Can you work these out from the model? Positions are in its coordinate system, mm. A direction names the side the tool comes from. Give positions to 0.01 mm unless a question says otherwise; leave off trailing zeros. Loops run counter-clockwise (first coordinate to the right, second up) from the corner with the lowest first, then second, coordinate; pieces in that order, holes last. Notation, with made-up numbers: M 73.25,6 L 115.25,6 A25 cw 115.25,26 Z; hole C -13,-23.5 d6. An arc over 180 degrees is marked long. Answer as a JSON object with one key per item and string values.
```python
from build123d import *

# Parameters (mm, degrees)
CROQUIS1_W                = 30
CROQUIS1_H                = 30
SALIENTE_EXTRUIR1_DEPTH   = 3
CROQUIS2_W                = 15
CROQUIS2_H                = 30
SALIENTE_EXTRUIR3_DEPTH   = 3
SALIENTE_EXTRUIR3_2_DEPTH = 3
CROQUIS3_W                = 30
CROQUIS3_H                = 30
SALIENTE_EXTRUIR4_DEPTH   = 3
SALIENTE_EXTRUIR5_DEPTH   = 3
CORTAR_EXTRUIR1_DEPTH     = 6
SALIENTE_EXTRUIR8_DEPTH   = 11
CROQUIS7_W                = 30
CROQUIS7_H                = 3.175
CORTAR_EXTRUIR3_DEPTH     = 18.542
CROQUIS9_W                = 60
CROQUIS9_H                = 0.175
SALIENTE_EXTRUIR9_DEPTH   = 11
CROQUIS10_W               = 90
CROQUIS10_H               = 5
CORTAR_EXTRUIR5_DEPTH     = 93
CROQUIS11_W               = 30
CROQUIS11_H               = 3.175
SALIENTE_EXTRUIR10_DEPTH  = 11
CROQUIS12_W               = 60
CROQUIS12_H               = 0.175
CORTAR_EXTRUIR6_DEPTH     = 11
CROQUIS14_W               = 30
CROQUIS14_H               = 6.35
CORTAR_EXTRUIR8_DEPTH     = 19.812
CROQUIS15_W               = 60
CROQUIS15_H               = 6.315381445
SALIENTE_EXTRUIR14_DEPTH  = 6
CROQUIS16_W               = 6.35
CROQUIS16_H               = 30
CORTAR_EXTRUIR9_DEPTH     = 10
CROQUIS17_W               = 3.35
CROQUIS17_H               = 60
SALIENTE_EXTRUIR15_DEPTH  = 6


with BuildPart() as part:
    # Croquis1 → Saliente-Extruir1 (new body)
    with BuildSketch(Plane(origin=(0, 0, 0), x_dir=(1, 0, 0), z_dir=(0, 1, 0))):
        Rectangle(CROQUIS1_W, CROQUIS1_H)
    extrude(amount=SALIENTE_EXTRUIR1_DEPTH)



with BuildPart() as body_2:
    # Croquis2 → Saliente-Extruir3 (new body)
    with BuildSketch(Plane(origin=(0, 3, 0), x_dir=(1, 0, 0), z_dir=(0, 1, 0))):
        with Locations((-22.5, -30)):
            Rectangle(CROQUIS2_W, CROQUIS2_H)
    extrude(amount=-SALIENTE_EXTRUIR3_DEPTH)


with BuildPart() as body_3:
    # Croquis2 → Saliente-Extruir3 2 (new body)
    with BuildSketch(Plane(origin=(0, 3, 0), x_dir=(1, 0, 0), z_dir=(0, 1, 0))):
        with Locations((22.5, -30)):
            Rectangle(CROQUIS2_W, CROQUIS2_H)
    extrude(amount=-SALIENTE_EXTRUIR3_2_DEPTH)


with BuildPart() as part_1:
    add(part.part)

    add(body_2.part)  # Saliente-Extruir4 merges body 2

    add(body_3.part)  # Saliente-Extruir4 merges body 3
    # Croquis3 → Saliente-Extruir4 (add)
    with BuildSketch(Plane(origin=(0, 3, 0), x_dir=(1, 0, 0), z_dir=(0, 1, 0))):
        with Locations((0, -30)):
            Rectangle(CROQUIS3_W, CROQUIS3_H)
    extrude(amount=-SALIENTE_EXTRUIR4_DEPTH)

    # Croquis4 → Saliente-Extruir5 (add)
    with BuildSketch(Plane(origin=(0, 3, 0), x_dir=(1, 0, 0), z_dir=(0, 1, 0))):
        Polygon((-30, 0), (-45, 0), (-45, -60), (45, -60), (45, 0), (30, 0), (30, 30), (-30, 30), align=None)
    extrude(amount=SALIENTE_EXTRUIR5_DEPTH)

    # Croquis5 → Cortar-Extruir1 (cut)
    with BuildSketch(Plane(origin=(0, 0, 0), x_dir=(-1, 0, 0), z_dir=(0, -1, 0))):
        Polygon((30, -45), (30, -15), (15, -15), (15, 15), (-15, 15), (-15, -15), (-30, -15), (-30, -45), align=None)
    extrude(amount=-CORTAR_EXTRUIR1_DEPTH, mode=Mode.SUBTRACT)

    # Croquis6 → Saliente-Extruir8 (add)
    with BuildSketch(Plane(origin=(0, 3, 0), x_dir=(-1, 0, 0), z_dir=(0, -1, 0))):
        with BuildLine():
            Line((37.5, 0), (45, 0))
            Line((45, 0), (45, -60))
            Line((45, -60), (-45, -60))
            Line((-45, -60), (-45, 0))
            Line((-45, 0), (-37.5, 0))
            ThreePointArc((-37.5, 0), (-32.196699141, 2.196699141), (-30, 7.5))
            Line((-30, 7.5), (-30, 30))
            Line((-30, 30), (30, 30))
            Line((30, 30), (30, 7.5))
            ThreePointArc((30, 7.5), (32.196699141, 2.196699141), (37.5, 0))
        make_face()
        Polygon((15, 15), (15, -15), (30, -15), (30, -45), (-30, -45), (-30, -15), (-15, -15), (-15, 15), align=None, mode=Mode.SUBTRACT)
    extrude(amount=-SALIENTE_EXTRUIR8_DEPTH)

    # Croquis7 → Cortar-Extruir3 (cut)
    with BuildSketch(Plane(origin=(0, 14, 0), x_dir=(1, 0, 0), z_dir=(0, 1, 0))):
        with Locations((0, 16.5875)):
            Rectangle(CROQUIS7_W, CROQUIS7_H)
    extrude(amount=-CORTAR_EXTRUIR3_DEPTH, mode=Mode.SUBTRACT)

    # Croquis9 → Saliente-Extruir9 (add)
    with BuildSketch(Plane(origin=(0, 14, 0), x_dir=(1, 0, 0), z_dir=(0, 1, 0))):
        with Locations((0, 30.0875)):
            Rectangle(CROQUIS9_W, CROQUIS9_H)
    extrude(amount=-SALIENTE_EXTRUIR9_DEPTH)

    # Croquis10 → Cortar-Extruir5 (cut)
    with BuildSketch(Plane.XY.offset(60)):
        with Locations((0, 5.5)):
            Rectangle(CROQUIS10_W, CROQUIS10_H)
    extrude(amount=-CORTAR_EXTRUIR5_DEPTH, mode=Mode.SUBTRACT)

    # Croquis11 → Saliente-Extruir10 (add)
    with BuildSketch(Plane(origin=(0, 14, 0), x_dir=(1, 0, 0), z_dir=(0, 1, 0))):
        with Locations((0, 16.5875)):
            Rectangle(CROQUIS11_W, CROQUIS11_H)
    extrude(amount=-SALIENTE_EXTRUIR10_DEPTH)

    # Croquis12 → Cortar-Extruir6 (cut)
    with BuildSketch(Plane(origin=(0, 14, 0), x_dir=(1, 0, 0), z_dir=(0, 1, 0))):
        with Locations((0, 30.0875)):
            Rectangle(CROQUIS12_W, CROQUIS12_H)
    extrude(amount=-CORTAR_EXTRUIR6_DEPTH, mode=Mode.SUBTRACT)

    # Croquis14 → Cortar-Extruir8 (cut)
    with BuildSketch(Plane(origin=(0, 14, 0), x_dir=(1, 0, 0), z_dir=(0, 1, 0))):
        with Locations((0, 18.175)):
            Rectangle(CROQUIS14_W, CROQUIS14_H)
    extrude(amount=-CORTAR_EXTRUIR8_DEPTH, mode=Mode.SUBTRACT)

    # Croquis15 → Saliente-Extruir14 (add)
    with BuildSketch(Plane(origin=(0, 14, 0), x_dir=(1, 0, 0), z_dir=(0, 1, 0))):
        with Locations((0, 30.192309278)):
            Rectangle(CROQUIS15_W, CROQUIS15_H)
    extrude(amount=-SALIENTE_EXTRUIR14_DEPTH)

    # Croquis16 → Cortar-Extruir9 (cut)
    with BuildSketch(Plane(origin=(0, 14, 0), x_dir=(1, 0, 0), z_dir=(0, 1, 0))):
        with Locations((-33.175, -30)):
            Rectangle(CROQUIS16_W, CROQUIS16_H)
        with Locations((33.175, -30)):
            Rectangle(CROQUIS16_W, CROQUIS16_H)
    extrude(amount=-CORTAR_EXTRUIR9_DEPTH, mode=Mode.SUBTRACT)

    # Croquis17 → Saliente-Extruir15 (add)
    with BuildSketch(Plane(origin=(0, 14, 0), x_dir=(1, 0, 0), z_dir=(0, 1, 0))):
        with Locations((-46.675, -30)):
            Rectangle(CROQUIS17_W, CROQUIS17_H)
        with Locations((46.675, -30)):
            Rectangle(CROQUIS17_W, CROQUIS17_H)
    extrude(amount=-SALIENTE_EXTRUIR15_DEPTH)


solid = part_1.part
```
1) Please list where these lines run through material, in increasing order: line 1 along Z through (x, y) = (-21, 12.1); line 2 along Z through (x, y) = (-1.5, 12.25); line 3 along X through (y, z) = (11.4, 13.5). Write a range as from..to.
Answer list:
{"line 1": "-33.35..15, 45..60", "line 2": "-33.35..-21.35, 45..60", "line 3": "-48.35..-15, 15..48.35"}
2) If we mould it in two halves opening along X, with no side actions, what happens to faces 5 (the flat face through (36.35, 11, 30)), 6 (the cylindrical face through (-32.139, 10.958, -2.255)), 7 (the flat face through (-22, 8, 13))? For each: +X half, -X half, draft (parallel to the pull), parting line (faces both ways), or undercut.
Answer list:
{"face 5": "undercut", "face 6": "-X half", "face 7": "draft"}
3) Will these pins go through, and if not, where does the flat tip stop? pin 1 Ø1.8 at (y, z) = (11.5, -25.5) entering from -X; pin 2 Ø3 at (x, y) = (45.5, 11) entering from -Z; pin 3 Ø1.8 at (y, z) = (10.5, -4) entering from +X; pin 4 Ø4 at (x, z) = (27, 42) entering from +Y (3 decimals).
Answer list:
{"pin 1": "x = -30", "pin 2": "z = 0", "pin 3": "x = 31.43", "pin 4": "through"}
4) Suppose I cut it at C-C, the plane y = 9.7. Write out the boundary of the cut face in (x, z).
Answer list:
{"outline": "M -48.35,0 L -37.5,0 A7.5 cw -30,-7.5 L -30,-33.35 L 30,-33.35 L 30,-7.5 A7.5 cw 37.5,0 L 48.35,0 L 48.35,60 L -48.35,60 Z; hole M -36.35,15 L -15,15 L -15,-21.35 L 15,-21.35 L 15,15 L 36.35,15 L 36.35,45 L -36.35,45 Z"}
5) For faces 1 (the flat face through (-36.35, 11, 30)), 2 (the flat face through (30, 11, -20)), 3 (the flat face through (-48.35, 11, 30)), 4 (the flat face through (-43, 11, 0)), which set-ups out of +Z, -Z, +X, -X, +Y, -Y let a thin tool reach every point of the face, with its end or its side?
Answer list:
{"face 1": "+Y, -Y", "face 2": "-Z, +X, +Y, -Y", "face 3": "+Z, -Z, -X, +Y, -Y", "face 4": "-Z, -X, +Y, -Y"}
6) Suppose I cut it at D-D, the plane z = -23. Write out the boundary of the cut face in (x, y), and give its area (3 significant figures).
Answer list:
{"outline": "M -30,8 L 30,8 L 30,14 L -30,14 Z", "area": "360 mm^2"}
7) Suppose I cut it at A-A, the plane z = 25. Write out the boundary of the cut face in (x, y), and give its area (3 significant figures).
Answer list:
{"outline": "M -48.35,8 L -36.35,8 L -36.35,14 L -48.35,14 Z; M 36.35,8 L 48.35,8 L 48.35,14 L 36.35,14 Z", "area": "144 mm^2"}
8) Suppose I cut it at B-B, the plane x = -31.5. Write out the boundary of the cut face in (y, z), and give its area (3 significant figures).
Answer list:
{"outline": "M 8,-3 L 14,-3 L 14,15 L 8,15 Z; M 8,45 L 14,45 L 14,60 L 8,60 Z", "area": "198 mm^2"}
